```python
from build123d import *

# Parameters (mm, degrees)
BOSS_EXTRU_1_DEPTH      = 11.5
ESQUISSE2_W             = 115
ESQUISSE2_H             = 21
BOSS_EXTRU_2_DEPTH      = 11.5
ENL_V_MAT_EXTRU_1_DEPTH = 8.5
ESQUISSE4_R             = 47.5
ENL_V_MAT_EXTRU_2_DEPTH = 148.618596389
D_GAGEMENT_M31_D        = 3.4


with BuildPart() as part:
    # Esquisse1 → Boss.-Extru.1 (new body)
    with BuildSketch(Plane.XY):
        with BuildLine():
            Line((57.5, 0), (-57.5, 0))
            Line((-57.5, 0), (-57.5, 76.5))
            ThreePointArc((-57.5, 76.5), (0, 134), (57.5, 76.5))
            Line((57.5, 76.5), (57.5, 0))
        make_face()
    extrude(amount=BOSS_EXTRU_1_DEPTH)

    # Esquisse2 → Boss.-Extru.2 (add)
    with BuildSketch(Plane.XY.offset(11.5)):
        with Locations((0, 10.5)):
            Rectangle(ESQUISSE2_W, ESQUISSE2_H)
    extrude(amount=BOSS_EXTRU_2_DEPTH)

    # Esquisse3 → Enlèv. mat.-Extru.1 (cut)
    with BuildSketch(Plane.XY.offset(11.5)):
        with BuildLine():
            Line((-54.5, 21), (-54.5, 76.5))
            ThreePointArc((-54.5, 76.5), (0, 131), (54.5, 76.5))
            Line((54.5, 76.5), (54.5, 21))
            Line((54.5, 21), (-54.5, 21))
        make_face()
    extrude(amount=-ENL_V_MAT_EXTRU_1_DEPTH, mode=Mode.SUBTRACT)

    # Esquisse4 → Enlèv. mat.-Extru.2 (cut, through all)
    with BuildSketch(Plane(origin=(0, 0, 0), x_dir=(-1, 0, 0), z_dir=(0, 0, -1))):
        with Locations((0, 76.5)):
            Circle(ESQUISSE4_R)
    extrude(amount=-ENL_V_MAT_EXTRU_2_DEPTH, mode=Mode.SUBTRACT)

    # Dégagement M31 (through all)
    with Locations(Plane(origin=(0, 0, 0), x_dir=(-1, 0, 0), z_dir=(0, 0, -1))):
        with Locations((-43.835096885, 102.566919286), (44.492162743, 101.428847837), (-0.657065858, 25.504232877)):
            Hole(D_GAGEMENT_M31_D / 2)


solid = part.part
```
Here's how the part is built. I have some questions about the finished solid (model axes, mm). A direction names the side the tool comes from. Give positions to 0.01 mm unless a question says otherwise; leave off trailing zeros. Write each loop counter-clockwise with the first axis right and the second up, starting at its lowest first coordinate (ties: lowest second). Pieces come first, ordered by that corner, then holes. Notation, with made-up numbers: M 0.25,-30 L 44.25,-30 A27 ccw 44.25,8 Z; hole C -38,-10 d3. An arc over 180 degrees is marked long. Put each result on its own line as item: value. Start each with the question number.
Item 1: If we section it at B-B, the plane z = 6.5: Write out the boundary of the cut face in (x, y).
Item 2: Will this pin go through, and if not, where does the flat tip stop? pin 1 (4.5 mm diameter, centred on x = -44.49, y = 101.43, fed in from +Z).
Item 3: If we section it at D-D, the plane z = 14.75: Write out the boundary of the cut face in (x, y).
Item 4: I need wall thicknesses on L1, parallel to X at y = 53, z = 9.25; L2, parallel to Y at x = -18, z = 15.25; L3, parallel to X at y = 86.5, z = 9.25. Which ranges of each line are inside material? Lowest first, please. Write a range as from..to.
Item 5: If we section it at C-C, the plane y = 51.5: Write out the boundary of the cut face in (x, z), then the cut area to 3 significant figures.
Item 6: On a 3-axis mill with a long thin cutter (end or side, diameter ignored), from which of +Z, -Z, +X, -X, +Y, -Y can I reach the whole of each face in a straight line? I mean faces 4 (the cylindrical face through (-1.198, 130.987, 7.31)), 5 (the flat face through (0, 132, 11.5)), 6 (the cylindrical face through (-43.71, 99.92, 1.52)). Say none if no direction works.
Item 7: If we section it at A-A, the plane x = 35.5: Write out the boundary of the cut face in (y, z), then the cut area to 3 significant figures.
Item 8: Thinking about a two-plate mould opening in X: for faces 1 (the flat face through (1, 23, 0)), 2 (the cylindrical face through (-1.264, 133.986, 5.67)), 3 (the cylindrical face through (6.184, 123.596, 1.479)), which applies, +X half, -X half, draft (parallel to the pull), parting line (faces both ways), or undercut?
Values:
1. outline: M -57.5,0 L 57.5,0 L 57.5,76.5 A57.5 ccw -57.5,76.5 Z; hole M -54.5,21 L 54.5,21 L 54.5,76.5 A54.5 ccw -54.5,76.5 Z
2. pin 1: z = 3
3. outline: M -57.5,0 L 57.5,0 L 57.5,21 L -57.5,21 Z
4. L1: -57.5..-54.5, 54.5..57.5
4. L2: 0..21
4. L3: -56.62..-53.57, 53.57..56.62
5. outline: M -57.5,0 L -40.39,0 L -40.39,3 L -54.5,3 L -54.5,11.5 L -57.5,11.5 Z; M 40.39,0 L 57.5,0 L 57.5,11.5 L 54.5,11.5 L 54.5,3 L 40.39,3 Z
5. area: 154 mm²
6. face 4: +Z
6. face 5: +Z, +X, -X, +Y
6. face 6: +Z, -Z
7. outline: M 0,0 L 44.94,0 L 44.94,3 L 21,3 L 21,23 L 0,23 Z; M 108.06,0 L 121.73,0 L 121.73,11.5 L 117.85,11.5 L 117.85,3 L 108.06,3 Z
7. area: 629 mm²
8. face 1: draft
8. face 2: parting line
8. face 3: undercut
